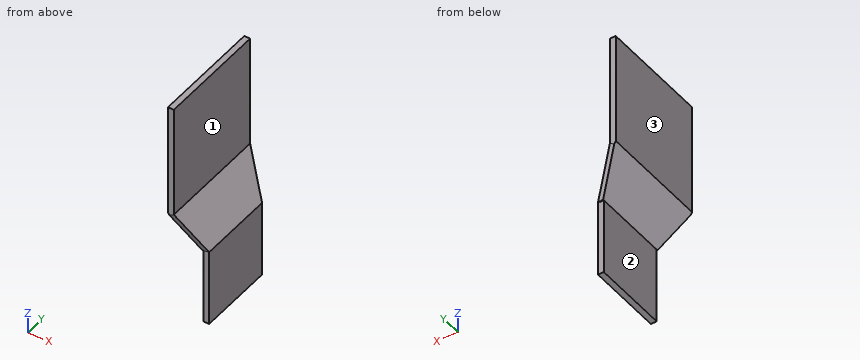
from build123d import *

# Parameters (mm, degrees)
F0_W     = 95
F0_H     = 95
F1_DEPTH = 5
F2_W     = 5
F2_H     = 65
F3_DEPTH = 95
F5_DEPTH = 25.4
F6_W     = 14.558809
F6_H     = 65
F7_DEPTH = 25.4


with BuildPart() as f1:
    # F0 (on Right) → F1 (new body)
    with BuildSketch(Plane.YZ):
        Rectangle(F0_W, F0_H)
    extrude(amount=F1_DEPTH)

    # F2 (on face) → F3 (join, through all)
    with BuildSketch(Plane.XZ.offset(47.5)):
        Polygon((25, -82.141016), (5, -47.5), (0, -47.5), (20, -82.141016), align=None)
        with Locations((22.5, -114.641016)):
            Rectangle(F2_W, F2_H)
    extrude(amount=-F3_DEPTH)

    # F4 (on face) → F5 (cut)
    with BuildSketch(Plane(origin=(-16.818103, 0, -9.709936), x_dir=(0, 1, 0), z_dir=(0.866025, 0, 0.5))):
        Polygon((-32.941191, -83.636207), (-47.5, -43.636207), (-47.5, -83.636207), align=None)
        Polygon((47.5, -83.636207), (47.5, -43.636207), (32.941191, -83.636207), align=None)
    extrude(amount=-F5_DEPTH, mode=Mode.SUBTRACT)

    # F6 (on face) → F7 (cut)
    with BuildSketch(Plane.YZ.offset(25)):
        with Locations((-40.220596, -114.641016)):
            Rectangle(F6_W, F6_H)
        with Locations((40.220596, -114.641016)):
            Rectangle(F6_W, F6_H)
    extrude(amount=-F7_DEPTH, mode=Mode.SUBTRACT)


solid = f1.part
The model under review builds one solid part; all positions refer to its coordinate system, in mm. Face numbers are marked on the shaded views. A direction names the side the tool comes from. Give positions to 0.01 mm unless a question says otherwise; leave off trailing zeros. Write each loop counter-clockwise with the first axis right and the second up, starting at its lowest first coordinate (ties: lowest second). Pieces come first, ordered by that corner, then holes.
1. Wall thickness on L1, parallel to X at y = -6.5, z = -8.5; L2, parallel to X at y = -21, z = -107.5; L3, parallel to Y at x = 23.5, z = -122: over which ranges is each line inside the solid? List them lowest first.
2. Add section A-A, the plane y = 3. Write out the cut boundary in (x, z).
3. Tool access review of the marked faces 1, 2 and 3: name each direction out of +Z, -Z, +X, -X, +Y, -Y from which nothing blocks a thin tool from reaching the whole face with its end or side.
4. Add section D-D, the plane x = 12. Write out the cut boundary in (y, z), plus the area to 3 significant figures.
5. Add section B-B, the plane z = -35.5. Write out the cut boundary in (x, y), plus the area to 3 significant figures.
6. Add section C-C, the plane x = 22.5. Write out the cut boundary in (y, z), plus the area to 3 significant figures.
7. For P1, Ø5.5, axis at x = 23.5, z = -123, coming from the -Y side; P2, Ø12, axis at y = 33.5, z = -39, coming from the +X side; P3, Ø6, axis at x = 5, y = 2, coming from the -Z side, all flat-tipped, find the tip position at first contact; note any pin that passes through.
Worked answers:
1. L1: x = 0 to 5
1. L2: x = 20 to 25
1. L3: y = -32.94 to 32.94
2. outline: (0, -47.5) - (20, -82.14) - (20, -147.14) - (25, -147.14) - (25, -82.14) - (5, -47.5) - (5, 47.5) - (0, 47.5) - close
3. face 1: +Z, +X, +Y, -Y
3. face 2: -Z, -X, +Y, -Y
3. face 3: +Z, -Z, -X, +Y, -Y
4. outline: (-42.4, -59.62) - (-39.67, -68.28) - (39.67, -68.28) - (42.4, -59.62) - close
4. area: 711 mm2
5. outline: (0, -47.5) - (5, -47.5) - (5, 47.5) - (0, 47.5) - close
5. area: 475 mm2
6. outline: (-34.76, -77.81) - (-33.4, -82.14) - (-32.94, -82.14) - (-32.94, -147.14) - (32.94, -147.14) - (32.94, -82.14) - (33.4, -82.14) - (34.76, -77.81) - close
6. area: 4,580 mm2
7. P1: stops at y = -32.94
7. P2: stops at x = 5
7. P3: stops at z = -61.36
